```python
from build123d import *

# Parameters (mm, degrees)
MODEL_R                 = 1.5
MODEL_W                 = 10
MODEL_H                 = 3
MODEL_W_2               = 3
MODEL_H_2               = 10
SALIENTE_EXTRUIR1_DEPTH = 3


with BuildPart() as part:
    # Model → Saliente-Extruir1 (new body)
    with BuildSketch(Plane.XY):
        with BuildLine():
            Line((-32.374234998, -40.258280816), (-32.374234998, 79.347619184))
            ThreePointArc((-32.374234998, 79.347619184), (-29.44530281, 86.418686996), (-22.374234998, 89.347619184))
            Line((-22.374234998, 89.347619184), (27.629122048, 89.347619184))
            ThreePointArc((27.629122048, 89.347619184), (30.675210948, 100.014701803), (38.63501695, 107.741719184))
            ThreePointArc((38.63501695, 107.741719184), (35.575059813, 98.684501141), (37.629122048, 89.347619184))
            Line((37.629122048, 89.347619184), (92.301279094, 89.347619184))
            ThreePointArc((92.301279094, 89.347619184), (99.372346906, 86.418686996), (102.301279094, 79.347619184))
            Line((102.301279094, 79.347619184), (102.301279094, -40.258280816))
            ThreePointArc((102.301279094, -40.258280816), (99.372346906, -47.329348628), (92.301279094, -50.258280816))
            Line((92.301279094, -50.258280816), (-22.374234998, -50.258280816))
            ThreePointArc((-22.374234998, -50.258280816), (-29.44530281, -47.329348628), (-32.374234998, -40.258280816))
        make_face()
        with Locations((67.080084989, -14.999118146)):
            Circle(MODEL_R, mode=Mode.SUBTRACT)
        with Locations((2.884992575, -15.037151741)):
            Circle(MODEL_R, mode=Mode.SUBTRACT)
        with Locations((2.884992575, 56.088341611)):
            Circle(MODEL_R, mode=Mode.SUBTRACT)
        with Locations((67.080084989, 56.088341611)):
            Circle(MODEL_R, mode=Mode.SUBTRACT)
        Polygon((43.960184493, -45.18534075), (43.960184493, -42.18534075), (53.960179079, -42.17493485), (53.960179079, -45.18534075), align=None, mode=Mode.SUBTRACT)
        with Locations((20.960165002, -43.68534075)):
            Rectangle(MODEL_W, MODEL_H, mode=Mode.SUBTRACT)
        Polygon((-0.287033943, 68.061018129), (-9.087685043, 59.260369229), (-25.611384998, 75.784069184), (-16.810734998, 84.584719184), align=None, mode=Mode.SUBTRACT)
        Polygon((78.959502691, 59.128875015), (95.576512855, 75.745885675), (86.737677959, 84.584720308), (70.120668893, 67.967710748), align=None, mode=Mode.SUBTRACT)
        Polygon((-25.611384913, -34.694730812), (-16.810686053, -43.495431871), (-0.28698502, -26.971730838), (-9.087686285, -18.171028474), align=None, mode=Mode.SUBTRACT)
        Polygon((86.737728061, -43.495431849), (95.538379094, -34.694780816), (79.014679094, -18.171080816), (70.214029117, -26.971730793), align=None, mode=Mode.SUBTRACT)
        with Locations((92.48239949, 43.571870396)):
            Rectangle(MODEL_W_2, MODEL_H_2, mode=Mode.SUBTRACT)
        with Locations((92.48239949, -2.520680527)):
            Rectangle(MODEL_W_2, MODEL_H_2, mode=Mode.SUBTRACT)
        with Locations((-25.18093295, -2.520680527)):
            Rectangle(MODEL_W_2, MODEL_H_2, mode=Mode.SUBTRACT)
        with Locations((-25.18093295, 43.571870396)):
            Rectangle(MODEL_W_2, MODEL_H_2, mode=Mode.SUBTRACT)
    extrude(amount=SALIENTE_EXTRUIR1_DEPTH)


solid = part.part
```
Geometry: final body of the model. Coordinates: model frame, mm. A direction names the side the tool comes from. Coordinates: 2 decimals unless noted, no trailing zeros. Order: outer loops, then holes, each group sorted by start corner. A loop starts at its lowest first (then second) coordinate and runs counter-clockwise, first axis right, second up.
Item 1: Access query for faces 1 (the face through (-4.63, -22.63, 1.48)), 2 (the face through (-29.367, -47.407, 1.479)). Directions: +Z, -Z, +X, -X, +Y, -Y. A direction counts if a zero-diameter tool reaches every point of the face in a straight line with its end or side. Return the directions, or none.
Answer:
face 1: +Z, -Z
face 2: +Z, -Z, -X, -Y
Item 2: Contact query for a flat-ended pin moving along its axis: P1, Ø1.5, axis at x = 63.5, z = 1.5, coming from the +Y side. Output: stop coordinate, or through.
Answer:
P1: stops at y = 89.35
Item 3: Section query C-C (y = 66). Output: boundary loops of the cut face in (x, z).
Answer:
outline: (-32.37, 0) - (-15.83, 0) - (-15.83, 3) - (-32.37, 3) - close; (-2.35, 0) - (72.09, 0) - (72.09, 3) - (-2.35, 3) - close; (85.83, 0) - (102.3, 0) - (102.3, 3) - (85.83, 3) - close
Item 4: Material intervals for line 1 along X through (y, z) = (-28, 1.8); line 2 along X through (y, z) = (-21, 1.35); line 3 along Y through (x, z) = (-24, 1.1), sorted ascending.
Answer:
line 1: x = -32.37 to -18.92, -1.32 to 71.24, 88.84 to 102.3
line 2: x = -32.37 to -11.92, -6.26 to 76.19, 81.84 to 102.3
line 3: y = -50.13 to -36.31, -33.08 to -7.52, 2.48 to 38.57, 48.57 to 74.17, 77.4 to 89.21
Item 5: Section query A-A (y = -1). Output: boundary loops of the cut face in (x, z), then the cut area to 3 significant figures.
Answer:
outline: (-32.37, 0) - (-26.68, 0) - (-26.68, 3) - (-32.37, 3) - close; (-23.68, 0) - (90.98, 0) - (90.98, 3) - (-23.68, 3) - close; (93.98, 0) - (102.3, 0) - (102.3, 3) - (93.98, 3) - close
area: 386 mm2
Item 6: Draft query along Y for faces 3 (the face through (-8.665, 76.439, 1.479)), 4 (the face through (99.4, -47.3, 1.5)), 5 (the face through (99.29, 86.5, 1.48)), 6 (the face through (-21.273, -39.033, 1.479)). Return one class per face: released by +Y, released by -Y, zero draft, split by the parting line, or undercut.
Answer:
face 3: undercut
face 4: released by -Y
face 5: released by +Y
face 6: undercut
Item 7: Section query D-D (z = 1.9). State how many separate pieces and enclosed holes the cut face has, then the cut area to 3 significant figures.
Answer:
separate pieces: 1
enclosed holes: 14
area: 17,400 mm2
Item 8: Section query B-B (x = 50.5). Output: boundary loops of the cut face in (y, z).
Answer:
outline: (-50.26, 0) - (-45.19, 0) - (-45.19, 3) - (-50.26, 3) - close; (-42.18, 0) - (89.35, 0) - (89.35, 3) - (-42.18, 3) - close
